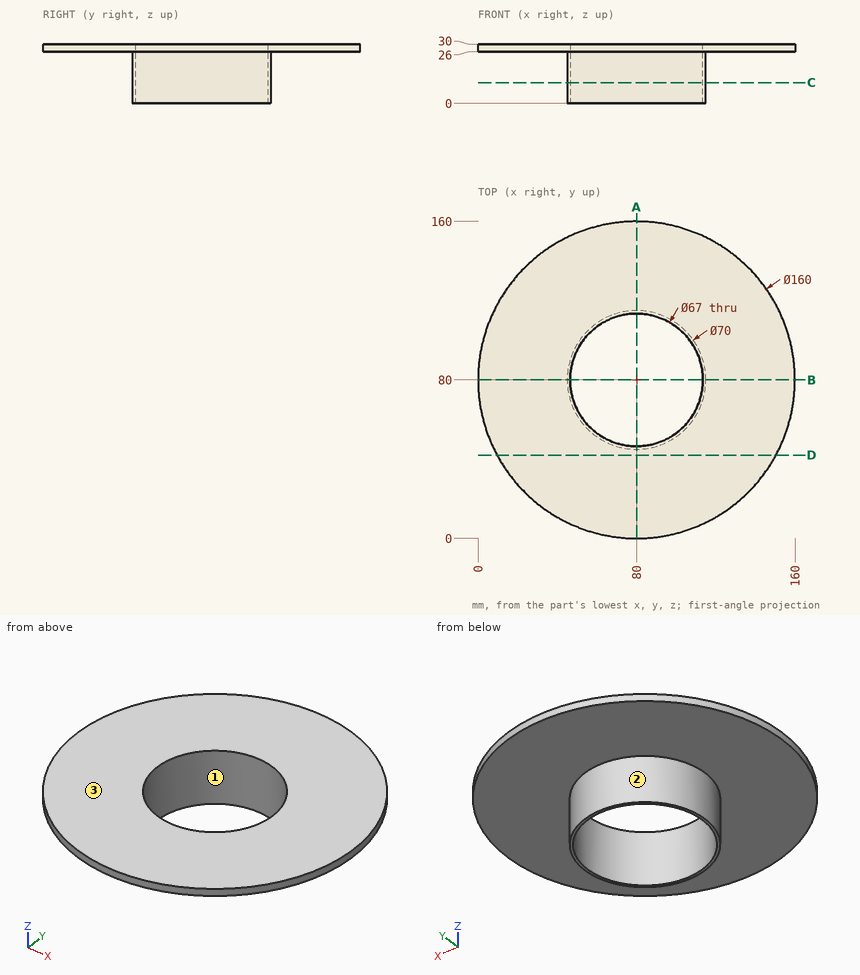
Geometry check sheet. Reference: drawing and pictorial views, mm from the part's lowest x, y, z. Round coordinates to 2 decimals unless told otherwise and drop trailing zeros. Loops run counter-clockwise (first coordinate to the right, second up) from the corner with the lowest first, then second, coordinate; pieces in that order, holes last. Notation, with made-up numbers: (85, 17.25) -> (90, 17.25) arc R15 ccw to (90, 22.25) -> close; hole circle Ø1 at (57, 78). An arc over 180 degrees is marked (long way). Answer as a JSON object with one key per item and string values. Group by question number.
Item 1: Thickness scan on line 1 along Y through (x, z) = (80, 22); line 2 along Z through (x, y) = (76, 10); line 3 along Y through (x, z) = (101, 24). Record the ranges inside material, lowest first.
Item 2: Cross-section at C-C, the plane z = 10.5. Record the cut outline in (x, y), plus the area to 3 significant figures.
Item 3: Depth check by flat-ended pin: pin 1 Ø1 at (x, z) = (78, 24.5) entering from -Y; pin 2 Ø2 at (x, z) = (95, 19.5) entering from +Y; pin 3 Ø6 at (x, y) = (31.5, 90) entering from -Z. Enter the tip coordinate at first touch or a pass-through.
Item 4: Cross-section at D-D, the plane y = 42. Record the cut outline in (x, z).
Item 5: Cross-section at A-A, the plane x = 80. Record the cut outline in (y, z), plus the area to 3 significant figures.
Item 6: Release check for a two-part mould opening along X. For the marked faces 1, 2 and 3 record: pulls with the +X half, pulls with the -X half, needs draft (parallel to the pull), parting line crosses it, or undercut.
Determined:
{
 "1": {"line 1": "y = 45 to 46.5, 113.5 to 115", "line 2": "z = 26 to 30", "line 3": "y = 52 to 53.9, 106.1 to 108"},
 "2": {"outline": "circle Ø70 at (80, 80); hole circle Ø67 at (80, 80)", "area": "323 mm²"},
 "3": {"pin 1": "stops at y = 45.03", "pin 2": "stops at y = 112.08", "pin 3": "stops at z = 26"},
 "4": {"outline": "(9.6, 26) -> (150.4, 26) -> (150.4, 30) -> (9.6, 30) -> close"},
 "5": {"outline": "(0, 26) -> (45, 26) -> (45, 0) -> (46.5, 0) -> (46.5, 30) -> (0, 30) -> close; (113.5, 0) -> (115, 0) -> (115, 26) -> (160, 26) -> (160, 30) -> (113.5, 30) -> close", "area": "450 mm²"},
 "6": {"face 1": "undercut", "face 2": "parting line crosses it", "face 3": "needs draft"}
}
